Check sheet for the modelled part. Datum: model origin and axes. Units: mm. Face numbers are marked on the shaded views. A direction names the side the tool comes from. Give positions to 0.01 mm unless a question says otherwise; leave off trailing zeros. Write each loop counter-clockwise with the first axis right and the second up, starting at its lowest first coordinate (ties: lowest second). Pieces come first, ordered by that corner, then holes. Notation, with made-up numbers: (-12.5, 82) -> (15.5, 82) arc R8 cw to (15.5, 97) -> close; hole circle Ø5 at (-4, 77.5). An arc over 180 degrees is marked (long way). Use a Markdown table: item, result. Add a question column.
1. Cross-section at B-B (z = -21.5). Enter the section's corners in (x, y), then the cut area to 3 significant figures.
2. Gauge pin test, flat ends, axial feed: P1, Ø5, axis at x = -25, z = -9.5, coming from the -Y side; P2, Ø1.5, axis at x = 14.5, z = 6.5, coming from the +Y side; P3, Ø12, axis at y = 19.5, z = 12, coming from the +X side; P4, Ø12, axis at x = -34.5, y = 14, coming from the +Z side. Record the tip position at first contact, or that the pin passes through.
3. Cross-section at D-D (x = -40.5). Enter the section's corners in (y, z).
4. Scan lines: probe 1 along X at (y, z) = (27.5, 0.5); probe 2 along Z at (x, y) = (21, 27); probe 3 along Z at (x, y) = (3.5, 2). Record each from-to range of solid material in increasing order. Write a range as [from, to].
5. Cross-section at A-A (y = 20). Enter the section's corners in (x, z), then the cut area to 3 significant figures.
6. Set-up check for the marked faces 1, 2 and 3: record each of +Z, -Z, +X, -X, +Y, -Y from which the full face is reachable in a straight line by a thin tool's end or side.
7. Cross-section at C-C (x = -19). Enter the section's corners in (y, z), then the cut area to 3 significant figures.
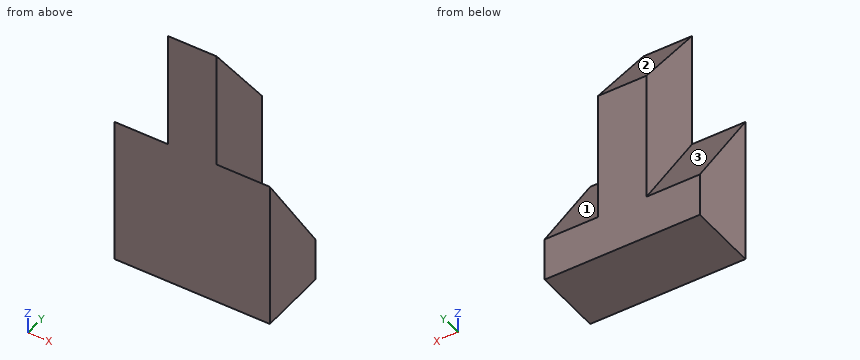
from build123d import *

# Parameters (mm, degrees)
F0_W      = 44.45
F0_H      = 38.1
F1_DEPTH  = 25.4
F2_DEPTH  = 56.388
F3_DEPTH  = 85.09
F6_DEPTH  = 29.21
F7_DEPTH  = 29.21
F8_DEPTH  = 64.516
F10_DEPTH = 25.4
F11_DEPTH = 25.4


with BuildPart() as f1:
    # F0 (on Top) → F1 (new body)
    with BuildSketch(Plane.XY):
        with Locations((-37.1782257403, 19.05)):
            Rectangle(F0_W, F0_H)
    extrude(amount=F1_DEPTH)

    # F2 (add): a face of the model
    f2_faces = [f1.faces().sort_by_distance(p)[0] for p in [
        (-37.1782257403, 19.05, 0),
    ]]
    extrude(f2_faces, amount=F2_DEPTH)

    # F3 (add): a face of the model
    f3_faces = [f1.faces().sort_by_distance(p)[0] for p in [
        (-59.4032257403, 19.05, -15.494),
    ]]
    extrude(f3_faces, amount=-F3_DEPTH)

    # F5 (on face) → F6 (cut)
    with BuildSketch(Plane.YZ.offset(25.6867742597)):
        Polygon((0, 25.4), (38.1, -32.4071533978), (38.1, 25.4), align=None)
    extrude(amount=-F6_DEPTH, mode=Mode.SUBTRACT)

    # F4 (on face) → F7 (cut)
    with BuildSketch(Plane(origin=(-59.4032257403, 0, 0), x_dir=(0, -1, 0), z_dir=(-1, 0, 0))):
        Polygon((-38.1, 25.4), (-38.1, -32.3631092906), (0, 25.4), align=None)
    extrude(amount=-F7_DEPTH, mode=Mode.SUBTRACT)

    # F8 (add): a face of the model
    f8_faces = [f1.faces().sort_by_distance(p)[0] for p in [
        (-16.8582257403, 19.05, 25.4),
    ]]
    extrude(f8_faces, amount=F8_DEPTH)

    # F9 (on face) → F10 (cut)
    with BuildSketch(Plane(origin=(-30.1932257403, 0, 0), x_dir=(0, -1, 0), z_dir=(-1, 0, 0))):
        Polygon((-38.1, 89.916), (-38.1, 39.8104563355), (0, 89.916), align=None)
    extrude(amount=-F10_DEPTH, mode=Mode.SUBTRACT)

    # F11 (cut): a face of the model
    f11_faces = [f1.faces().sort_by_distance(p)[0] for p in [
        (-4.7932257403, 25.4, 73.2141521118),
    ]]
    extrude(f11_faces, amount=-F11_DEPTH, mode=Mode.SUBTRACT)


solid = f1.part
Worked answers:
| question | item | result |
|---|---|---|
| 1 | outline | (-59.4, 0) -> (25.69, 0) -> (25.69, 30.91) -> (-3.52, 30.91) -> (-3.52, 38.1) -> (-30.19, 38.1) -> (-30.19, 30.93) -> (-59.4, 30.93) -> close |
| 1 | area | 2,820 mm² |
| 2 | P1 | stops at y = 0 |
| 2 | P2 | stops at y = 12.95 |
| 2 | P3 | stops at x = -3.52 |
| 2 | P4 | stops at z = 77 |
| 3 | outline | (0, -56.39) -> (38.1, -56.39) -> (38.1, -32.36) -> (0, 25.4) -> close |
| 4 | probe 1 | x = [-30.19, -3.52] |
| 4 | probe 2 | z = [-56.39, -15.57] |
| 4 | probe 3 | z = [-56.39, 22.37] |
| 5 | outline | (-59.4, -56.39) -> (25.69, -56.39) -> (25.69, -4.94) -> (-3.52, -4.94) -> (-3.52, 63.61) -> (-30.19, 63.61) -> (-30.19, -4.92) -> (-59.4, -4.92) -> close |
| 5 | area | 6,210 mm² |
| 6 | face 1 | +Z, +X, +Y |
| 6 | face 2 | +Z, +X, -X, +Y |
| 6 | face 3 | +Z, -X, +Y |
| 7 | outline | (0, -56.39) -> (38.1, -56.39) -> (38.1, 39.81) -> (0, 89.92) -> close |
| 7 | area | 4,620 mm² |
